Check sheet for the modelled part. Datum: model origin and axes. Units: mm. A direction names the side the tool comes from. Give positions to 0.01 mm unless a question says otherwise; leave off trailing zeros. Loops run counter-clockwise (first coordinate to the right, second up) from the corner with the lowest first, then second, coordinate; pieces in that order, holes last. Notation, with made-up numbers: (34.5, -28) -> (71.5, -28) arc R20 cw to (71.5, -18) -> close; hole circle Ø4 at (79.25, 67.25). An arc over 180 degrees is marked (long way). Write each question's results on one line, items separated by ' | '. Start each with the question number.
1. Cross-section at B-B on x = -61. Record the boundary of the cut face in (y, z), and give its area (3 significant figures).
2. Material ranges on L1, parallel to X at y = 19, z = 49; L2, parallel to Y at x = -48.5, z = 24.5; L3, parallel to Z at x = -85.5, y = 19.5, recorded low to high. Write a range as from..to.
3. Cross-section at A-A on y = 36. Record the boundary of the cut face in (x, z), and give its area (3 significant figures).
4. Cross-section at C-C on z = 74.5. Record the boundary of the cut face in (x, y), and give its area (3 significant figures).
5. Tool access check on faces 1 (the face through (-21.981, 4.93, 92.594)), 2 (the face through (-65, 20, 125)), 3 (the face through (-56, 25, 110)). Record the directions out of +Z, -Z, +X, -X, +Y, -Y that give a thin tool (end or side, any length) a straight path to the whole face; none if there is none.
6. Gauge pin test, flat ends, axial feed: pin 1 Ø1 at (y, z) = (9, 13) entering from -X; pin 2 Ø4 at (x, z) = (-33, -62.5) entering from +Y; pin 3 Ø5 at (y, z) = (4.5, 36) entering from -X; pin 4 Ø8 at (x, y) = (-55, 7.5) entering from -Z. Record the tip position at first contact, or that the pin passes through.
7. Mould release check, pull along Z, two halves, no side actions. Record for faces 4 (the face through (-64.635, 19.72, -1.208)), 5 (the face through (10.3, 20, -1)), 6 (the face through (-19.7, 5, 48)), 7 (the face through (-10.771, 24.79, -52.926)): +Z half, -Z half, draft (parallel to the pull), parting line (faces both ways), or undercut.
8. Cross-section at D-D on y = 4. Record the boundary of the cut face in (x, z), and give its area (3 significant figures).
Autodesk Inventor part; units mm, degrees
ref_plane "YZ Plane" through (0, 0, 0) normal (1, 0, 0) x (0, 1, 0)
ref_plane "XZ Plane" through (0, 0, 0) normal (0, 1, 0) x (-1, 0, 0)
ref_plane "XY Plane" through (0, 0, 0) normal (0, 0, 1) x (1, 0, 0)
sketch "Sketch1" plane through (0, 0, 0) normal (0, 1, 0) x (-1, 0, 0)
  line L0 (137.5, 125) -> (-10.3, 125)
  line L1 (-10.3, 125) -> (-10.3, -131)
  line L2 (-10.3, -131) -> (137.5, -131)
  line L3 (137.5, -131) -> (137.5, 125)
  line L4 (137.5, 125) -> (-10.3, -131)
  point P0 (0, 0)
  dimension "d0" = 256
  dimension "d1" = 147.8
  dimension "d7" = 30
extrude "Extrusion1" add sketch "Sketch1" along normal blind 40 contours L4 L1 L0
sketch "Sketch2" plane through (0, 40, 0) normal (0, 1, 0) x (1, 0, 0)
  line L0 (-137.5, -125) -> (10.3, -125) construction
  line L1 (10.3, -125) -> (10.3, 131) construction
  line L2 (10.3, 131) -> (-137.5, -125) construction
  line L3 (-137.5, -125) -> (10.3, -125) construction
  line L4 (10.3, -125) -> (10.3, 131) construction
  line L5 (10.3, 131) -> (-137.5, -125) construction
  line L6 (-111.5194, -110) -> (-4.7, -110)
  line L7 (-4.7, -110) -> (-4.7, 75.0187)
  line L8 (-4.7, 75.0187) -> (-111.5194, -110)
  point P0 (0, 0)
  dimension "d4" = 15
extrude "Extrusion2" cut sketch "Sketch2" against normal blind 30
sketch "Sketch3" plane through (0, 10, 0) normal (0, 1, 0) x (1, 0, 0)
  line L0 (-4.7, 75.0187) -> (-4.7, -110) construction
  line L1 (-111.5194, -110) -> (-4.7, 75.0187) construction
  line L2 (-4.7, -110) -> (-111.5194, -110) construction
  point P0 (0, 0)
sketch "Sketch4" plane through (0, 10, 0) normal (0, 1, 0) x (1, 0, 0)
  line L0 (-4.7, 75.0187) -> (-4.7, -110) construction
  line L1 (-111.5194, -110) -> (-4.7, 75.0187) construction
  line L2 (-4.7, -110) -> (-111.5194, -110) construction
  line L3 (-4.7, 75.0187) -> (-4.7, -110) construction
  line L4 (-111.5194, -110) -> (-4.7, 75.0187) construction
  line L5 (-4.7, -110) -> (-111.5194, -110) construction
  line L6 (-19.7, 19.0374) -> (-19.7, -95)
  line L7 (-19.7, -95) -> (-85.5388, -95)
  line L8 (-85.5388, -95) -> (-19.7, 19.0374)
  point P0 (0, 0)
  dimension "d9" = 15
extrude "Extrusion3" cut sketch "Sketch4" against normal blind 30
fillet "Fillet2" radius 8 6 edges at (-4.7, 25, -75.0187) (-111.5194, 25, 110) (-4.7, 25, 110) (-19.7, 5, 95) (-85.5388, 5, 95) (-19.7, 5, -19.0374)
properties part number "StaninaOpora.iam" material "Aluminum 6061"
Geometry says:
1) outline: (0, -7.5) -> (40, -7.5) -> (40, 22.5) -> (10, 22.5) -> (10, 52.5) -> (0, 52.5) -> close; (0, 95) -> (10, 95) -> (10, 110) -> (40, 110) -> (40, 125) -> (0, 125) -> close | area: 2,250 mm^2
2) L1: -93.62..-76.3, -4.7..10.3 | L2: 0..10 | L3: 34.93..64.93, 110..125
3) outline: (-137.5, 125) -> (10.3, -131) -> (10.3, 125) -> close; hole (-104.59, 98) -> (-19.63, -49.16) arc R8 ccw to (-4.7, -45.16) -> (-4.7, 102) arc R8 ccw to (-12.7, 110) -> (-97.66, 110) arc R8 ccw to start | area: 9,250 mm^2
4) outline: (-108.34, 0) -> (-73.7, 0) -> (-73.7, 10) -> (-91.02, 10) -> (-91.02, 40) -> (-108.34, 40) -> close; (-19.7, 0) -> (10.3, 0) -> (10.3, 40) -> (-4.7, 40) -> (-4.7, 10) -> (-19.7, 10) -> close | area: 1,620 mm^2
5) face 1: +Y, -Y | face 2: +Z, +X, -X, +Y, -Y | face 3: +Y
6) pin 1: x = -73.13 | pin 2: through | pin 3: x = -87.56 | pin 4: z = -24.82
7) face 4: -Z half | face 5: draft | face 6: undercut | face 7: undercut
8) outline: (-137.5, 125) -> (10.3, -131) -> (10.3, 125) -> close; hole (-78.61, 83) -> (-34.63, 6.82) arc R8 ccw to (-19.7, 10.82) -> (-19.7, 87) arc R8 ccw to (-27.7, 95) -> (-71.68, 95) arc R8 ccw to start | area: 15,400 mm^2
